from build123d import *
from build123d.topology import SkipClean

# Parameters (mm, degrees)
SKETCH_3_R                       = 13.752444878
EXTRUDE_2_DEPTH                  = 5
CUT_EXTRUDE_2_DEPTH              = 21.081321676
FILLET_1_R                       = 0.48
PATTERN_CIRCULAR_1_COUNT         = 18
FILLET_1_OF_PATTERN_CIRCULAR_1_R = 0.48
SKETCH_4_R                       = 4.05
CUT_EXTRUDE_3_DEPTH              = 22.772520597
EXTRUDE_START                    = 5.7
SKETCH_5_R                       = 7
SKETCH_5_R_2                     = 4.05
EXTRUDE_3_DEPTH                  = 5.7
SKETCH_8_W                       = 1.2
SKETCH_8_H                       = 13.59826875


with BuildPart() as part:
    # Sketch 3 → Extrude 2 (new, symmetric)
    with BuildSketch(Plane.XY):
        Circle(SKETCH_3_R)
    extrude(amount=EXTRUDE_2_DEPTH, both=True)

    # Sketch 3_3 → Cut-Extrude 2 (cut, symmetric)
    with BuildSketch(Plane.XY):
        with BuildLine():
            Line((-1.597131903, 13.659389072), (-1.524613435, 13.039178578))
            ThreePointArc((-1.524613435, 13.039178578), (0, 11.682444878), (1.524613435, 13.039178578))
            Line((1.524613435, 13.039178578), (1.597131903, 13.659389072))
            ThreePointArc((1.597131903, 13.659389072), (0, 13.752444878), (-1.597131903, 13.659389072))
        make_face()
    cut_extrude_2 = extrude(amount=CUT_EXTRUDE_2_DEPTH, both=True, mode=Mode.SUBTRACT)

    # Fillet 1
    fillet_1_edges = [part.edges().sort_by_distance(p)[0] for p in [
        (-1.597131903, 13.659389072, 0),
        (1.597131903, 13.659389072, 0),
    ]]
    fillet(fillet_1_edges, radius=FILLET_1_R)

    # Pattern Circular 1: Cut-Extrude 2 ×18 about axis
    pattern_circular_1_axis = Axis((0, 0, 0), (0, 0, 1))
    for i in range(1, PATTERN_CIRCULAR_1_COUNT):
        add(cut_extrude_2.rotate(pattern_circular_1_axis, i * 360 / PATTERN_CIRCULAR_1_COUNT), mode=Mode.SUBTRACT)

    # Fillet 1 of Pattern Circular 1
    fillet_1_of_pattern_circular_1_edges = [part.edges().sort_by_distance(p)[0] for p in [
        (-6.172599272, 12.289375833, 0),
        (-3.170973145, 13.381878398, 0),
        (-10.00356007, 9.437082497, 0),
        (-7.556612032, 11.490315693, 0),
        (-12.627943888, 5.446537735, 0),
        (-11.030811985, 8.212851337, 0),
        (-13.729211304, 0.79906014, 0),
        (-13.174533215, 3.944795901, 0),
        (-13.174533215, -3.944795901, 0),
        (-13.729211304, -0.79906014, 0),
        (-11.030811985, -8.212851337, 0),
        (-12.627943888, -5.446537735, 0),
        (-7.556612032, -11.490315693, 0),
        (-10.00356007, -9.437082497, 0),
        (-3.170973145, -13.381878398, 0),
        (-6.172599272, -12.289375833, 0),
        (1.597131903, -13.659389072, 0),
        (-1.597131903, -13.659389072, 0),
        (6.172599272, -12.289375833, 0),
        (3.170973145, -13.381878398, 0),
        (10.00356007, -9.437082497, 0),
        (7.556612032, -11.490315693, 0),
        (12.627943888, -5.446537735, 0),
        (11.030811985, -8.212851337, 0),
        (13.729211304, -0.79906014, 0),
        (13.174533215, -3.944795901, 0),
        (13.174533215, 3.944795901, 0),
        (13.729211304, 0.79906014, 0),
        (11.030811985, 8.212851337, 0),
        (12.627943888, 5.446537735, 0),
        (7.556612032, 11.490315693, 0),
        (10.00356007, 9.437082497, 0),
        (3.170973145, 13.381878398, 0),
        (6.172599272, 12.289375833, 0),
    ]]
    fillet(fillet_1_of_pattern_circular_1_edges, radius=FILLET_1_OF_PATTERN_CIRCULAR_1_R)

    # Sketch 4 → Cut-Extrude 3 (cut, through all)
    with BuildSketch(Plane(origin=(0, 0, -5), x_dir=(-1, 0, 0), z_dir=(0, 0, -1))):
        Circle(SKETCH_4_R)
    extrude(amount=-CUT_EXTRUDE_3_DEPTH, mode=Mode.SUBTRACT)

    # Sketch 5 → Extrude 3 (add)
    with BuildSketch(Plane(origin=(0, 0, -5), x_dir=(-1, 0, 0), z_dir=(0, 0, -1)).offset(EXTRUDE_START)):
        with Locations(Location((0, 0, 0), (0, 0, 180))):
            Circle(SKETCH_5_R)
        Circle(SKETCH_5_R_2, mode=Mode.SUBTRACT)
    extrude(amount=-EXTRUDE_3_DEPTH)

    # Sketch 8 → M3x0.5 _ _ _ _1 (revolve, cut)
    with BuildSketch(Plane(origin=(0, 0, -7.85), x_dir=(0, 0, -1), z_dir=(1, 0, 0))):
        with Locations((0.6, 6.799134375)):
            Rectangle(SKETCH_8_W, SKETCH_8_H)
    revolve(axis=Axis((0, -6.35, -7.85), (0, 1, 0)), mode=Mode.SUBTRACT)

    # Sketch 9 → Revolve 1 (revolve)
    with SkipClean():  # the faces are left unmerged after this step: merging them gives an invalid solid
        with BuildSketch(Plane(origin=(0, 0, 0), x_dir=(0, 0, -1), z_dir=(1, 0, 0))):
            with BuildLine():
                Line((-5.7, 16.112561362), (-5.7, 4.05))
                Line((-5.7, 4.05), (-5, 4.05))
                Line((-5, 4.05), (-5, 14.592692947))
                ThreePointArc((-5, 14.592692947), (-5.183409788, 15.429352974), (-5.7, 16.112561362))
            make_face()
            with BuildLine():
                Line((5, 4.05), (5, 14.592692947))
                ThreePointArc((5, 14.592692947), (5.183409788, 15.429352974), (5.7, 16.112561362))
                Line((5.7, 16.112561362), (5.7, 4.05))
                Line((5.7, 4.05), (5, 4.05))
            make_face()
        revolve(axis=Axis((0, 0, 0), (0, 0, 1)))


solid = part.part
Model file for the job. Use its own axes, mm. A direction names the side the tool comes from. Coordinates: 2 decimals unless noted, no trailing zeros. Order: outer loops, then holes, each group sorted by start corner. A loop starts at its lowest first (then second) coordinate and runs counter-clockwise, first axis right, second up. Notation, with made-up numbers: M 69.25,-20.5 L 81.25,-20.5 A25 ccw 81.25,9.5 Z; hole C -9.5,37.25 d10. An arc over 180 degrees is marked long. Return JSON: item names as keys, results as strings.
1. Flat gauge pins, fed straight in: pin 1 (3 mm diameter, centred on x = 3, z = 0.5, fed in from -Y); pin 2 (1.5 mm diameter, centred on x = -7.5, z = 1.5, fed in from -Y); pin 3 (13 mm diameter, centred on x = 0, y = 0, fed in from +Z); pin 4 (3 mm diameter, centred on x = 0, z = -7.85, fed in from -Y). Where does each tip first touch, or does it go through?
Ans:
{"pin 1": "y = -13.6", "pin 2": "y = -11.98", "pin 3": "z = 5.7", "pin 4": "y = -7"}
2. Saw through at A-A (z = -8). Give the cut face in (x, y), and give its area (3 significant figures).
Ans:
{"outline": "M -1.19,3.87 L -1.19,6.9 A7 ccw long 1.19,6.9 L 1.19,3.87 A4.05 cw long Z", "area": "95.3 mm^2"}
3. Pull direction Y, two halves, no side cores. Call faces 4 (the face through (7, 3, -5.7)), 5 (the face through (6.466, 2.681, -8.235)), 6 (the face through (-10.133, 5.814, 0.07)): +Y half, -Y half, draft (parallel to the pull), parting line (faces both ways), or undercut.
Ans:
{"face 4": "draft", "face 5": "parting line", "face 6": "undercut"}
4. Tool access for faces 1 (the face through (0.031, -11.683, 0.07)), 2 (the face through (12, -2, 5)), 3 (the face through (-0.031, 11.683, 0.07)): list every direction of +Z, -Z, +X, -X, +Y, -Y with a clear straight run to the whole face (end or side of a thin tool).
Ans:
{"face 1": "-Y", "face 2": "none", "face 3": "+Y"}
5. Drill centre lines: probe 1 along Z at (x, y) = (0, 5.9); probe 2 along X at (y, z) = (0, -2.25); probe 3 along Z at (x, y) = (-12.5, -8.5). Where is each one in solid material? Low to high.
Ans:
{"probe 1": "-10.7 to -9.05, -6.65 to 5.7", "probe 2": "-13.75 to -4.05, 4.05 to 13.75", "probe 3": "-5.7 to -5.07, 5.07 to 5.7"}
